For this review, take the finished solid that the model builds, in its own axes (mm). Face numbers are marked on the shaded views. Round coordinates to 2 decimals unless told otherwise and drop trailing zeros. Order: outer loops, then holes, each group sorted by start corner. A loop starts at its lowest first (then second) coordinate and runs counter-clockwise, first axis right, second up. Notation, with made-up numbers: M -10.75,37.5 L 26.25,37.5 A32 ccw 26.25,70.5 Z; hole C 67,0.25 d7. An arc over 180 degrees is marked long. Put each result on its own line as item: value.
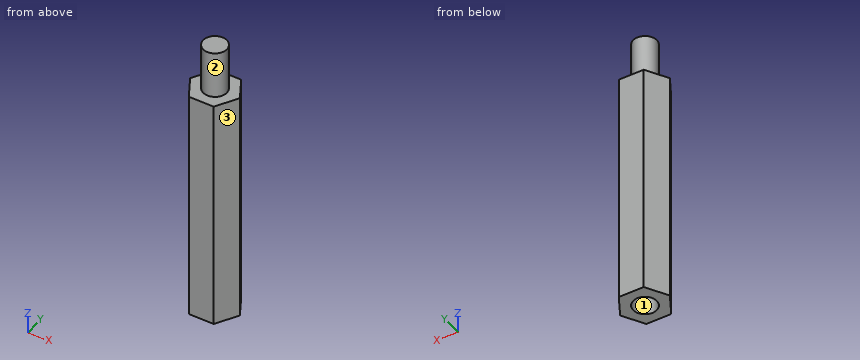
from build123d import *

# Parameters (mm, degrees)
PAD_DEPTH    = 30
SKETCH001_R  = 1.5
PAD001_DEPTH = 6
SKETCH002_R  = 1.5
POCKET_DEPTH = 15


with BuildPart() as part:
    # Sketch → Pad (new body)
    with BuildSketch(Plane.XY):
        Polygon((1.587713, -2.75), (3.175426, 0), (1.587713, 2.75), (-1.587713, 2.75), (-3.175426, 0), (-1.587713, -2.75), align=None)
    extrude(amount=PAD_DEPTH)

    # Sketch001 (on Face8 of Pad) → Pad001 (join)
    with BuildSketch(Plane.XY.offset(30)):
        Circle(SKETCH001_R)
    extrude(amount=PAD001_DEPTH)

    # Sketch002 (on Face4 of Pad001) → Pocket (cut)
    with BuildSketch(Plane(origin=(0, 0, 0), x_dir=(1, 0, 0), z_dir=(0, 0, -1))):
        Circle(SKETCH002_R)
    extrude(amount=-POCKET_DEPTH, mode=Mode.SUBTRACT)


solid = part.part
(1) Add section A-A on z = 4. Give the boundary of the cut face in (x, y), then the cut area to 3 significant figures.
A:
outline: M -3.18,0 L -1.59,-2.75 L 1.59,-2.75 L 3.18,0 L 1.59,2.75 L -1.59,2.75 Z; hole C 0,0 d3
area: 19.1 mm2
(2) To check wall thickness, follow L1, parallel to Y at x = 0, z = 4.75; L2, parallel to Z at x = 1.25, y = 1.15; L3, parallel to Z at x = 0, y = -0.05. State the ranges of each line that lie inside material, in increasing order.
A:
L1: y = -2.75 to -1.5, 1.5 to 2.75
L2: z = 0 to 30
L3: z = 15 to 36
(3) Add section D-D on z = 17.5. Give the boundary of the cut face in (x, y).
A:
outline: M -3.18,0 L -1.59,-2.75 L 1.59,-2.75 L 3.18,0 L 1.59,2.75 L -1.59,2.75 Z
(4) Draft analysis for pull direction Y (two halves, no side actions). For the marked faces 1, 2 and 3, state which applies: released by +Y, released by -Y, zero draft, split by the parting line, or undercut.
A:
face 1: undercut
face 2: split by the parting line
face 3: released by -Y
(5) Add section B-B on x = 0. Give the boundary of the cut face in (y, z), then the cut area to 3 significant figures.
A:
outline: M -2.75,0 L -1.5,0 L -1.5,15 L 1.5,15 L 1.5,0 L 2.75,0 L 2.75,30 L 1.5,30 L 1.5,36 L -1.5,36 L -1.5,30 L -2.75,30 Z
area: 138 mm2
(6) Add section C-C on y = -1.2. Give the boundary of the cut face in (x, z).
A:
outline: M -2.48,0 L -0.9,0 L -0.9,15 L 0.9,15 L 0.9,0 L 2.48,0 L 2.48,30 L 0.9,30 L 0.9,36 L -0.9,36 L -0.9,30 L -2.48,30 Z
(7) Insertion check: pin 1 Ø1.5 at (x, y) = (0, 0.5) entering from -Z; pin 2 Ø2 at (x, z) = (2, 31.5) entering from -Y; pin 3 Ø1.5 at (y, z) = (0.5, 11) entering from -X. Each pin has a flat end and moves straight along its axis. Give the tip position at first contact, or say it passes through.
A:
pin 1: stops at z = 15
pin 2: stops at y = -1.12
pin 3: stops at x = -3.18
